from build123d import *

# Parameters (mm, degrees)
SKETCH1_W                                           = 98
SKETCH1_H                                           = 60
BOSS_EXTRUDE1_DEPTH                                 = 10
CBORE_FOR_M5_HEX_SOCKET_HEAD_CAP_SCREW1_D           = 5.5
CBORE_FOR_M5_HEX_SOCKET_HEAD_CAP_SCREW1_CBORE_D     = 10
CBORE_FOR_M5_HEX_SOCKET_HEAD_CAP_SCREW1_CBORE_DEPTH = 5.4


with BuildPart() as part:
    # Sketch1 → Boss-Extrude1 (new body)
    with BuildSketch(Plane(origin=(0, 0, 0), x_dir=(1, 0, 0), z_dir=(0, 1, 0))):
        Rectangle(SKETCH1_W, SKETCH1_H)
    extrude(amount=BOSS_EXTRUDE1_DEPTH)

    # CBORE for M5 Hex Socket Head Cap Screw1 (through all)
    with Locations(Plane(origin=(0, 0, 0), x_dir=(-1, 0, 0), z_dir=(0, -1, 0))):
        with Locations((6, 17), (-17, 17), (-17, -17), (6, -17)):
            CounterBoreHole(CBORE_FOR_M5_HEX_SOCKET_HEAD_CAP_SCREW1_D / 2, CBORE_FOR_M5_HEX_SOCKET_HEAD_CAP_SCREW1_CBORE_D / 2, CBORE_FOR_M5_HEX_SOCKET_HEAD_CAP_SCREW1_CBORE_DEPTH)


solid = part.part
Source: CAD feature listing. Evaluate the final solid. Frame: model axes, mm. A direction names the side the tool comes from. Round coordinates to 2 decimals unless told otherwise and drop trailing zeros. Write each loop counter-clockwise with the first axis right and the second up, starting at its lowest first coordinate (ties: lowest second). Pieces come first, ordered by that corner, then holes. Notation, with made-up numbers: M 20.5,53.25 L 66.5,53.25 A17 ccw 66.5,58.25 Z; hole C -26,49 d1. An arc over 180 degrees is marked long. One line per item, written item: value. Start each with the question number.
Item 1: Set-up query: faces 1 (the flat face through (-1, 0, 0)), 2 (the cylindrical face through (18.08, 2.66, 21.88)). Return all of +Z, -Z, +X, -X, +Y, -Y with unobstructed straight access to the full face (end or side cutting, diameter ignored); none if empty.
Item 2: Section query B-B (z = -17). Return the cut outline in (x, y), plus the area to 3 significant figures.
Item 3: Section query A-A (x = -6). Return the cut outline in (y, z).
Item 4: Ray query, L1, parallel to X at y = 1.95, z = 17; L2, parallel to Z at x = -6, y = 1.95; L3, parallel to X at y = 8.85, z = -17. Return the intervals inside material, ascending. Write a range as from..to.
Item 5: Mould query, pull axis Z, two halves, no side actions, for faces 3 (the cylindrical face through (-3.38, 7.73, 16.17)), 4 (the flat face through (49, 5, 0)), 5 (the flat face through (-8.2, 5.4, -14.8)), 6 (the flat face through (-1, 5, -30)). Classes: pulls with the +Z half, pulls with the -Z half, needs draft (parallel to the pull), parting line crosses it, or undercut.
Item 6: Pin query (flat end, axial travel): pin 1 (5 mm diameter, centred on x = -7.5, z = -15.5, fed in from -Y). Return the tip coordinate at first contact, or that it passes through.
Result set:
1. face 1: +Z, -Z, +X, -X, -Y
1. face 2: -Y
2. outline: M -49,0 L -11,0 L -11,5.4 L -8.75,5.4 L -8.75,10 L -49,10 Z; M -3.25,5.4 L -1,5.4 L -1,0 L 12,0 L 12,5.4 L 14.25,5.4 L 14.25,10 L -3.25,10 Z; M 19.75,5.4 L 22,5.4 L 22,0 L 49,0 L 49,10 L 19.75,10 Z
2. area: 821 mm²
3. outline: M 0,-30 L 10,-30 L 10,-19.75 L 5.4,-19.75 L 5.4,-22 L 0,-22 Z; M 0,-12 L 5.4,-12 L 5.4,-14.25 L 10,-14.25 L 10,14.25 L 5.4,14.25 L 5.4,12 L 0,12 Z; M 0,22 L 5.4,22 L 5.4,19.75 L 10,19.75 L 10,30 L 0,30 Z
4. L1: x = -49..-11, -1..12, 22..49
4. L2: z = -30..-22, -12..12, 22..30
4. L3: x = -49..-8.75, -3.25..14.25, 19.75..49
5. face 3: undercut
5. face 4: needs draft
5. face 5: undercut
5. face 6: pulls with the -Z half
6. pin 1: stops at y = 5.4
